Can you work these out from the model? Positions are in its coordinate system, mm. Coordinates: 2 decimals unless noted, no trailing zeros. Order: outer loops, then holes, each group sorted by start corner. A loop starts at its lowest first (then second) coordinate and runs counter-clockwise, first axis right, second up. Notation, with made-up numbers: (12.25, -20) -> (47.25, -20) arc R11 cw to (47.25, -11) -> close; hole circle Ø7 at (75.5, 28). An arc over 180 degrees is marked (long way). Answer as a JSON object with one key per item and string values. Group by question number.
(1) I need wall thicknesses on line 1 (Y direction, x = 78.74, z = -1.95); line 2 (Y direction, x = -156.5, z = -3); line 3 (X direction, y = 4, z = -2.95). Which ranges of each line are inside material? Lowest first, please.
(2) I want a section at C-C, the plane z = -0.7. State how many separate pieces and enclosed holes the cut face has, plus the area to 3 significant figures.
(3) I want a section at B-B, the plane y = 120. List the corners of the cut face in (x, z) for me (3 decimals), plus the area to 3 significant figures.
(4) I want a section at D-D, the plane x = 143.5. List the corners of the cut face in (y, z) for me (3 decimals), plus the area to 3 significant figures.
(5) I want a section at A-A, the plane x = 70. List the corners of the cut face in (y, z) for me (3 decimals).
Autodesk Inventor part; units mm, degrees
ref_plane "YZ Plane" through (0, 0, 0) normal (1, 0, 0) x (0, 1, 0)
ref_plane "XZ Plane" through (0, 0, 0) normal (0, 1, 0) x (-1, 0, 0)
ref_plane "XY Plane" through (0, 0, 0) normal (0, 0, 1) x (1, 0, 0)
sketch "Sketch1" plane through (0, 0, 0) normal (0, 0, 1) x (1, 0, 0)
  circle A0 centre (0, 0) radius 136.271
  circle A1 centre (0, 0) radius 190.5
  dimension "d0" = 272.542
  dimension "d1" = 381
extrude "Extrusion1" add sketch "Sketch1" against normal blind 3.175
sketch "Sketch2" plane through (0, 0, 0) normal (0, 0, 1) x (1, 0, 0)
  circle A0 centre (0, 0) radius 157.48 construction
  circle A1 centre (-157.48, 0) radius 3.9687
  circle A2 centre (-78.74, -136.3817) radius 3.9687
  circle A3 centre (78.74, -136.3817) radius 3.9687
  circle A4 centre (157.48, 0) radius 3.9687
  circle A5 centre (78.74, 136.3817) radius 3.9687
  circle A6 centre (-78.74, 136.3817) radius 3.9687
  dimension "d6" = 314.96
  dimension "d7" = 7.9375
  dimension "d8" = 360
extrude "Extrusion2" cut sketch "Sketch2" against normal through all
sketch "Sketch3" plane through (0, 0, 0) normal (0, 0, 1) x (1, 0, 0)
  line L0 (0, 0) -> (0, -177.8) construction
  line L1 (0, 0) -> (177.8, 0) construction
  circle A0 centre (0, -177.8) radius 3.81
  circle A1 centre (153.9793, -88.9) radius 3.81
  circle A2 centre (153.9793, 88.9) radius 3.81
  circle A3 centre (0, 177.8) radius 3.81
  circle A4 centre (-153.9793, 88.9) radius 3.81
  circle A5 centre (-153.9793, -88.9) radius 3.81
  line L2 (0, 0) -> (0, -177.8) construction
  line L3 (0, 0) -> (177.8, 0) construction
  circle A6 centre (0, -177.8) radius 3.81
  circle A7 centre (153.9793, -88.9) radius 3.81
  circle A8 centre (153.9793, 88.9) radius 3.81
  circle A9 centre (0, 177.8) radius 3.81
  circle A10 centre (-153.9793, 88.9) radius 3.81
  circle A11 centre (-153.9793, -88.9) radius 3.81
  line L4 (0, 0) -> (0, -177.8) construction
  line L5 (0, 0) -> (177.8, 0) construction
  circle A12 centre (0, -177.8) radius 3.81
  circle A13 centre (153.9793, -88.9) radius 3.81
  circle A14 centre (153.9793, 88.9) radius 3.81
  circle A15 centre (0, 177.8) radius 3.81
  circle A16 centre (-153.9793, 88.9) radius 3.81
  circle A17 centre (-153.9793, -88.9) radius 3.81
  dimension "d13" = 177.8
  dimension "d14" = 90
  dimension "d15" = 7.62
  dimension "d16" = 360
  dimension "d19" = 177.8
  dimension "d20" = 90
  dimension "d21" = 7.62
  dimension "d22" = 360
  dimension "d25" = 177.8
  dimension "d26" = 90
  dimension "d27" = 7.62
  dimension "d28" = 360
extrude "Extrusion3" cut sketch "Sketch3" against normal through all
ref_plane "Work Plane1" through (0, 0, 0) normal (0, 0, 1) x (1, 0, 0)
sketch "Sketch4" plane through (0, 0, 0) normal (0, 0, 1) x (1, 0, 0)
  circle A0 centre (0, 0) radius 124.1061 construction
properties part number "Ring Gear Outer"
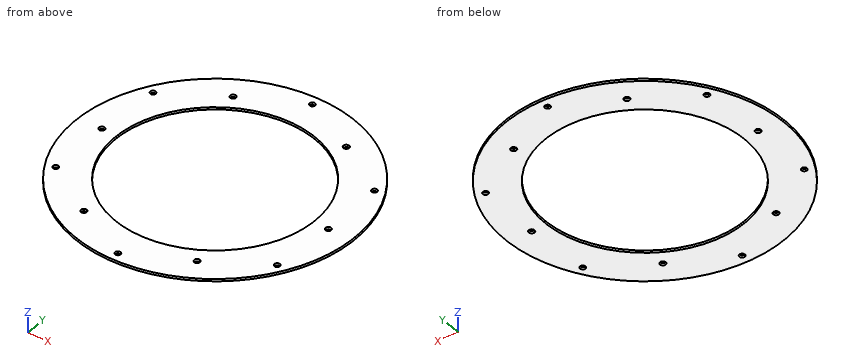
Computed values:
{
 "1": {"line 1": "y = -173.47 to -140.35, -132.41 to -111.22, 111.22 to 132.41, 140.35 to 173.47", "line 2": "y = -108.62 to -91.76, -86.04 to -3.85, 3.85 to 86.04, 91.76 to 108.62", "line 3": "x = -190.46 to -136.21, 136.21 to 190.46"},
 "2": {"separate pieces": "1", "enclosed holes": "13", "area": "55,100 mm2"},
 "3": {"outline": "(-147.954, -3.175) -> (-64.574, -3.175) -> (-64.574, 0) -> (-147.954, 0) -> close; (64.574, -3.175) -> (147.954, -3.175) -> (147.954, 0) -> (64.574, 0) -> close", "area": "529 mm2"},
 "4": {"outline": "(-125.292, -3.175) -> (125.292, -3.175) -> (125.292, 0) -> (-125.292, 0) -> close", "area": "796 mm2"},
 "5": {"outline": "(-177.173, -3.175) -> (-116.918, -3.175) -> (-116.918, 0) -> (-177.173, 0) -> close; (116.918, -3.175) -> (177.173, -3.175) -> (177.173, 0) -> (116.918, 0) -> close"}
}
